The model under review builds one solid part; all positions refer to its coordinate system, in mm. A direction names the side the tool comes from. Round coordinates to 2 decimals unless told otherwise and drop trailing zeros. Write each loop counter-clockwise with the first axis right and the second up, starting at its lowest first coordinate (ties: lowest second). Pieces come first, ordered by that corner, then holes. Notation, with made-up numbers: (-31.5, 34.5) -> (6.5, 34.5) arc R13 ccw to (6.5, 41.5) -> close; hole circle Ø11 at (-3.5, -30). An arc over 180 degrees is marked (long way). Return JSON: item names as keys, results as strings. Group by question number.
1. Clearance check with flat-ended pins moving along their axes: P1, Ø8, axis at y = 30, z = -2.5, coming from the -X side; P2, Ø0.6, axis at y = 33.5, z = -16.5, coming from the +X side; P3, Ø3.5, axis at x = 12.5, z = -12.5, coming from the -Y side; P4, Ø2, axis at y = 69, z = -1, coming from the -X side. State where each tip first meets the part, or that it passes through.
2. Mouldability with a two-part tool opening along X and no side actions: class faces 1 (the flat face through (-16.5, 41, 0)), 2 (the flat face through (7, 39, -17)), 3 (the flat face through (-13, 72.8, 13)) as pulls with the +X half, pulls with the -X half, needs draft (parallel to the pull), parting line crosses it, or undercut.
3. Tool access review of faces 4 (the cylindrical face through (14.483, 3.803, -12.24)), 5 (the flat face through (0, 66.5, 0)), 6 (the cylindrical face through (15, 40.6, -14.9)): name each direction out of +Z, -Z, +X, -X, +Y, -Y from which nothing blocks a thin tool from reaching the whole face with its end or side.
4. For line 1 along X through (y, z) = (77.5, -12.5); line 2 along X through (y, z) = (29, 3.5), list the stretches that pass through material, from the lowest coordinate up. Write a range as from..to.
5. Take a section at B-B, the plane x = 0. Write out the cut boundary in (y, z).
from build123d import *

# Parameters (mm, degrees)
SKETCH_1_W           = 34
SKETCH_1_H           = 34
EXTRUDE_1_DEPTH      = 80
FILLET_1_R           = 7
CUT_EXTRUDE_8_REACH  = 85.534
SKETCH_13_W          = 10
SKETCH_13_H          = 0.5
SKETCH_13_W_2        = 0.5
SKETCH_13_H_2        = 10
CHAMFER_1_SIZE       = 0.5
SKETCH_18_R          = 2
CUT_EXTRUDE_9_DEPTH  = 7.2
CHAMFER_2_SIZE       = 0.5
CUT_EXTRUDE_START    = -7.2
SKETCH_19_R          = 2
CUT_EXTRUDE_10_DEPTH = 7.2
CHAMFER_3_SIZE       = 0.5
SKETCH_20_R          = 12.5
EXTRUDE_2_DEPTH      = 1.5
CHAMFER_4_SIZE       = 0.5
SKETCH_21_R          = 7
SKETCH_21_R_2        = 1.5
CUT_EXTRUDE_11_DEPTH = 1.5
SKETCH_23_R          = 7
CUT_EXTRUDE_12_DEPTH = 13.5
CUT_EXTRUDE_START_2  = -80
SKETCH_10_W          = 10
SKETCH_10_H          = 0.5
CUT_EXTRUDE_4_DEPTH  = 80
SKETCH_12_W          = 0.5
SKETCH_12_H          = 10
CUT_EXTRUDE_5_DEPTH  = 80


with BuildPart() as part:
    # ｽｹｯﾁ1 → ﾎﾞｽ - 押し出し1 (new body)
    with BuildSketch(Plane(origin=(0, 0, 0), x_dir=(1, 0, 0), z_dir=(0, 1, 0))):
        Rectangle(SKETCH_1_W, SKETCH_1_H)
    extrude(amount=EXTRUDE_1_DEPTH)

    # ﾌｨﾚｯﾄ1
    fillet_1_edges = [part.edges().sort_by_distance(p)[0] for p in [
        (-17, 40, -17),
        (17, 40, -17),
        (17, 40, 17),
        (-17, 40, 17),
    ]]
    fillet(fillet_1_edges, radius=FILLET_1_R)

    # ｽｹｯﾁ13 → ｶｯﾄ - 押し出し8 (cut, up to next)
    with BuildSketch(Plane.XZ, mode=Mode.PRIVATE) as cut_extrude_8_sk1:
        with Locations((0, 16.75)):
            Rectangle(SKETCH_13_W, SKETCH_13_H)
    cut_extrude_8_tool1 = extrude(cut_extrude_8_sk1.sketch, amount=-CUT_EXTRUDE_8_REACH, mode=Mode.PRIVATE) & part.part
    # ｽｹｯﾁ13 → ｶｯﾄ - 押し出し8 (cut, up to next)
    with BuildSketch(Plane.XZ, mode=Mode.PRIVATE) as cut_extrude_8_sk2:
        with Locations((-16.75, 0)):
            Rectangle(SKETCH_13_W_2, SKETCH_13_H_2)
    cut_extrude_8_tool2 = extrude(cut_extrude_8_sk2.sketch, amount=-CUT_EXTRUDE_8_REACH, mode=Mode.PRIVATE) & part.part
    # ｽｹｯﾁ13 → ｶｯﾄ - 押し出し8 (cut, up to next)
    with BuildSketch(Plane.XZ, mode=Mode.PRIVATE) as cut_extrude_8_sk3:
        with Locations((0, -16.75)):
            Rectangle(SKETCH_13_W, SKETCH_13_H)
    cut_extrude_8_tool3 = extrude(cut_extrude_8_sk3.sketch, amount=-CUT_EXTRUDE_8_REACH, mode=Mode.PRIVATE) & part.part
    # ｽｹｯﾁ13 → ｶｯﾄ - 押し出し8 (cut, up to next)
    with BuildSketch(Plane.XZ, mode=Mode.PRIVATE) as cut_extrude_8_sk4:
        with Locations((16.75, 0)):
            Rectangle(SKETCH_13_W_2, SKETCH_13_H_2)
    cut_extrude_8_tool4 = extrude(cut_extrude_8_sk4.sketch, amount=-CUT_EXTRUDE_8_REACH, mode=Mode.PRIVATE) & part.part
    add(cut_extrude_8_tool1.solids().sort_by_distance((0, 0, 16.75))[0], mode=Mode.SUBTRACT)
    add(cut_extrude_8_tool2.solids().sort_by_distance((-16.75, 0, 0))[0], mode=Mode.SUBTRACT)
    add(cut_extrude_8_tool3.solids().sort_by_distance((0, 0, -16.75))[0], mode=Mode.SUBTRACT)
    add(cut_extrude_8_tool4.solids().sort_by_distance((16.75, 0, 0))[0], mode=Mode.SUBTRACT)

    # 面取り1
    chamfer_1_edges = [part.edges().sort_by_distance(p)[0] for p in [
        (-5, 40, 16.5),
        (5, 40, 16.5),
        (16.5, 40, 5),
        (16.5, 40, -5),
        (5, 40, -16.5),
        (-5, 40, -16.5),
        (-16.5, 40, -5),
        (-16.5, 40, 5),
    ]]
    chamfer(chamfer_1_edges, length=CHAMFER_1_SIZE - 0.0001)  # a hair under: the kernel refuses the full size

    # ｽｹｯﾁ18 → ｶｯﾄ - 押し出し9 (cut)
    with BuildSketch(Plane.XZ):
        with Locations(Location((12.5, -12.5, 0), (0, 0, 270))):
            Circle(SKETCH_18_R)
        with Locations(Location((-12.5, 12.5, 0), (0, 0, 270))):
            Circle(SKETCH_18_R)
    extrude(amount=-CUT_EXTRUDE_9_DEPTH, mode=Mode.SUBTRACT)

    # 面取り2
    chamfer_2_edges = [part.edges().sort_by_distance(p)[0] for p in [
        (12.5, 0, -10.5),
        (-12.5, 0, 14.5),
    ]]
    chamfer(chamfer_2_edges, length=CHAMFER_2_SIZE)

    # ｽｹｯﾁ19 → ｶｯﾄ - 押し出し10 (cut)
    with BuildSketch(Plane(origin=(0, 80, 0), x_dir=(1, 0, 0), z_dir=(0, 1, 0)).offset(CUT_EXTRUDE_START)):
        with Locations(Location((-12.5, -12.5, 0), (0, 0, 90))):
            Circle(SKETCH_19_R)
        with Locations(Location((-12.5, 12.5, 0), (0, 0, 270))):
            Circle(SKETCH_19_R)
        with Locations(Location((12.5, 12.5, 0), (0, 0, 90))):
            Circle(SKETCH_19_R)
        with Locations(Location((12.5, -12.5, 0), (0, 0, 270))):
            Circle(SKETCH_19_R)
    extrude(amount=CUT_EXTRUDE_10_DEPTH, mode=Mode.SUBTRACT)

    # 面取り3
    chamfer_3_edges = [part.edges().sort_by_distance(p)[0] for p in [
        (-12.5, 80, -14.5),
        (-12.5, 80, 14.5),
        (12.5, 80, -10.5),
        (12.5, 80, 10.5),
    ]]
    chamfer(chamfer_3_edges, length=CHAMFER_3_SIZE)

    # ｽｹｯﾁ20 → ﾎﾞｽ - 押し出し2 (add)
    with BuildSketch(Plane(origin=(0, 80, 0), x_dir=(1, 0, 0), z_dir=(0, 1, 0))):
        with Locations(Location((0, 0, 0), (0, 0, 270))):
            Circle(SKETCH_20_R)
    extrude(amount=EXTRUDE_2_DEPTH)

    # 面取り4
    chamfer_4_edges = [part.edges().sort_by_distance(p)[0] for p in [
        (0, 81.5, -12.5),
    ]]
    chamfer(chamfer_4_edges, length=CHAMFER_4_SIZE)

    # ｽｹｯﾁ21 → ｶｯﾄ - 押し出し11 (cut)
    with BuildSketch(Plane(origin=(0, 81.5, 0), x_dir=(1, 0, 0), z_dir=(0, 1, 0))):
        with Locations(Location((0, 0, 0), (0, 0, 270))):
            Circle(SKETCH_21_R)
        with Locations(Location((9.5, 0, 0), (0, 0, 270))):
            Circle(SKETCH_21_R_2)
        with Locations(Location((-9.5, 0, 0), (0, 0, 270))):
            Circle(SKETCH_21_R_2)
    extrude(amount=-CUT_EXTRUDE_11_DEPTH, mode=Mode.SUBTRACT)

    # ｽｹｯﾁ23 → ｶｯﾄ - 押し出し12 (cut)
    with BuildSketch(Plane(origin=(0, 80, 0), x_dir=(1, 0, 0), z_dir=(0, 1, 0))):
        with Locations(Location((0, 0, 0), (0, 0, 270))):
            Circle(SKETCH_23_R)
    extrude(amount=-CUT_EXTRUDE_12_DEPTH, mode=Mode.SUBTRACT)

    # ｽｹｯﾁ10 → ｶｯﾄ - 押し出し4 (cut)
    with BuildSketch(Plane.XZ.offset(CUT_EXTRUDE_START_2)):
        with Locations((0, -16.75)):
            Rectangle(SKETCH_10_W, SKETCH_10_H)
    extrude(amount=CUT_EXTRUDE_4_DEPTH, mode=Mode.SUBTRACT)

    # ｽｹｯﾁ12 → ｶｯﾄ - 押し出し5 (cut)
    with BuildSketch(Plane.XZ.offset(CUT_EXTRUDE_START_2)):
        with Locations((-16.75, 0)):
            Rectangle(SKETCH_12_W, SKETCH_12_H)
    extrude(amount=CUT_EXTRUDE_5_DEPTH, mode=Mode.SUBTRACT)


solid = part.part
Output:
{
 "1": {"P1": "stops at x = -17", "P2": "stops at x = 13.25", "P3": "stops at y = 7.2", "P4": "stops at x = -16.5"},
 "2": {"face 1": "pulls with the -X half", "face 2": "needs draft", "face 3": "undercut"},
 "3": {"face 4": "-Y", "face 5": "+Y", "face 6": "-Z, +X, +Y, -Y"},
 "4": {"line 1": "x = -16.54..-14.5, -10.5..10.5, 14.5..16.54", "line 2": "x = -16.5..16.5"},
 "5": {"outline": "(0, -16.5) -> (80, -16.5) -> (80, -12.5) -> (81, -12.5) -> (81.5, -12) -> (81.5, -7) -> (66.5, -7) -> (66.5, 7) -> (81.5, 7) -> (81.5, 12) -> (81, 12.5) -> (80, 12.5) -> (80, 16.5) -> (0, 16.5) -> close"}
}
